from build123d import *

# Parameters (mm, degrees)
SKETCH_1_W          = 20
SKETCH_1_H          = 12
SKETCH_1_R          = 1.6
SKETCH_1_R_2        = 2.1
EXTRUDE_1_DEPTH     = 5.3
EXTRUDE_2_DEPTH     = 1.5
SKETCH_1_5_R        = 1.6
EXTRUDE_3_DEPTH     = 4
EXTRUDE_START       = 5.3
EXTRUDE_4_DEPTH     = 4.5
SKETCH_2_R          = 0.9
SKETCH_2_R_2        = 0.7
CUT_EXTRUDE_1_DEPTH = 26.299011838
CUT_EXTRUDE_START   = 9.8
SKETCH_2_3_R        = 1.5
CUT_EXTRUDE_2_DEPTH = 8.8
SKETCH_2_4_R        = 1
CUT_EXTRUDE_3_DEPTH = 7.8
SKETCH_2_5_R        = 0.3
CUT_EXTRUDE_4_DEPTH = 6


with BuildPart() as part:
    # 草图1 → 凸台-拉伸1 (new body)
    with BuildSketch(Plane(origin=(0, 0, 0), x_dir=(1, 0, 0), z_dir=(0, 1, 0))):
        with Locations((10, -6)):
            Rectangle(SKETCH_1_W, SKETCH_1_H)
        with BuildLine():
            ThreePointArc((12.439835428, -3.613463312), (18.220575086, -7.370363498), (11.50515478, -5.81011348))
            ThreePointArc((11.50515478, -5.81011348), (7.454652656, -2.789434091), (12.439835428, -3.613463312))
        make_face(mode=Mode.SUBTRACT)
        with Locations(Location((7.678736094, -8.970584613, 0), (0, 0, 270))):
            Circle(SKETCH_1_R, mode=Mode.SUBTRACT)
        with Locations(Location((5, -6, 0), (0, 0, 270))):
            Circle(SKETCH_1_R_2, mode=Mode.SUBTRACT)
    extrude(amount=EXTRUDE_1_DEPTH)

    # 草图1<4> → 凸台-拉伸2 (add)
    with BuildSketch(Plane(origin=(0, 0, 0), x_dir=(1, 0, 0), z_dir=(0, 1, 0))):
        with BuildLine():
            ThreePointArc((11.50515478, -5.81011348), (11.779424914, -4.629636502), (12.439835428, -3.613463312))
            ThreePointArc((12.439835428, -3.613463312), (7.454652656, -2.789434091), (11.50515478, -5.81011348))
        make_face()
    extrude(amount=EXTRUDE_2_DEPTH)

    # 草图1<5> → 凸台-拉伸3 (add)
    with BuildSketch(Plane(origin=(0, 0, 0), x_dir=(1, 0, 0), z_dir=(0, 1, 0))):
        with Locations(Location((7.678736094, -8.970584613, 0), (0, 0, 270))):
            Circle(SKETCH_1_5_R)
    extrude(amount=EXTRUDE_3_DEPTH)

    # 草图1<6> → 凸台-拉伸4 (add)
    with BuildSketch(Plane(origin=(0, 0, 0), x_dir=(1, 0, 0), z_dir=(0, 1, 0)).offset(EXTRUDE_START)):
        with BuildLine():
            Line((7.958677072, 0), (0, 0))
            Line((0, 0), (0, -12))
            Line((0, -12), (5.925840657, -12))
            ThreePointArc((5.925840657, -12), (4.429268792, -10.270954659), (4.319841502, -7.986802561))
            ThreePointArc((4.319841502, -7.986802561), (3.000111311, -5.359340003), (5.600909971, -3.987810345))
            ThreePointArc((5.600909971, -3.987810345), (6.188678117, -1.644412009), (7.958677072, 0))
        make_face()
        with BuildLine():
            Line((20, 0), (11.735482653, 0))
            ThreePointArc((11.735482653, 0), (12.869036074, -0.819060885), (13.675372646, -1.961700559))
            ThreePointArc((13.675372646, -1.961700559), (18.910698319, -7.664012819), (11.171707216, -7.845717845))
            ThreePointArc((11.171707216, -7.845717845), (11.090844977, -7.871351024), (11.009487245, -7.895365208))
            ThreePointArc((11.009487245, -7.895365208), (10.945672327, -10.226422042), (9.43163153, -12))
            Line((9.43163153, -12), (20, -12))
            Line((20, -12), (20, 0))
        make_face()
    extrude(amount=EXTRUDE_4_DEPTH)

    # 草图2 → 切除-拉伸1 (cut, through all)
    with BuildSketch(Plane(origin=(0, 0, 0), x_dir=(1, 0, 0), z_dir=(0, 1, 0))):
        with Locations(Location((2.3, -2.214171161, 0), (0, 0, 270))):
            Circle(SKETCH_2_R)
        with Locations(Location((7.7, -9.785828839, 0), (0, 0, 313.840961576))):
            Circle(SKETCH_2_R)
        with Locations(Location((11.5, -1.5, 0), (0, 0, 171.097944201))):
            Circle(SKETCH_2_R_2)
        with Locations(Location((18.5, -10.5, 0), (0, 0, 270))):
            Circle(SKETCH_2_R_2)
        with Locations(Location((18.5, -1.5, 0), (0, 0, 270))):
            Circle(SKETCH_2_R_2)
        with Locations(Location((11.5, -10.5, 0), (0, 0, 132.232284036))):
            Circle(SKETCH_2_R_2)
    extrude(amount=CUT_EXTRUDE_1_DEPTH, mode=Mode.SUBTRACT)

    # 草图2<3> → 切除-拉伸2 (cut)
    with BuildSketch(Plane(origin=(0, 0, 0), x_dir=(1, 0, 0), z_dir=(0, 1, 0)).offset(CUT_EXTRUDE_START)):
        with Locations(Location((2.3, -2.214171161, 0), (0, 0, 270))):
            Circle(SKETCH_2_3_R)
        with Locations(Location((7.7, -9.785828839, 0), (0, 0, 270))):
            Circle(SKETCH_2_3_R)
    extrude(amount=-CUT_EXTRUDE_2_DEPTH, mode=Mode.SUBTRACT)

    # 草图2<4> → 切除-拉伸3 (cut)
    with BuildSketch(Plane(origin=(0, 0, 0), x_dir=(1, 0, 0), z_dir=(0, 1, 0)).offset(CUT_EXTRUDE_START)):
        with Locations((11.5, -1.5)):
            Circle(SKETCH_2_4_R)
        with Locations(Location((18.5, -10.5, 0), (0, 0, 270))):
            Circle(SKETCH_2_4_R)
        with Locations(Location((18.5, -1.5, 0), (0, 0, 270))):
            Circle(SKETCH_2_4_R)
        with Locations(Location((11.5, -10.5, 0), (0, 0, 270))):
            Circle(SKETCH_2_4_R)
    extrude(amount=-CUT_EXTRUDE_3_DEPTH, mode=Mode.SUBTRACT)

    # 草图2<5> → 切除-拉伸4 (cut)
    with BuildSketch(Plane(origin=(0, 0, 0), x_dir=(1, 0, 0), z_dir=(0, 1, 0)).offset(CUT_EXTRUDE_START)):
        with Locations(Location((1.5, -6, 0), (0, 0, 270))):
            Circle(SKETCH_2_5_R)
        with Locations(Location((16.5, -1.1, 0), (0, 0, 270))):
            Circle(SKETCH_2_5_R)
        with Locations(Location((15, -10.9, 0), (0, 0, 270))):
            Circle(SKETCH_2_5_R)
    extrude(amount=-CUT_EXTRUDE_4_DEPTH, mode=Mode.SUBTRACT)


solid = part.part
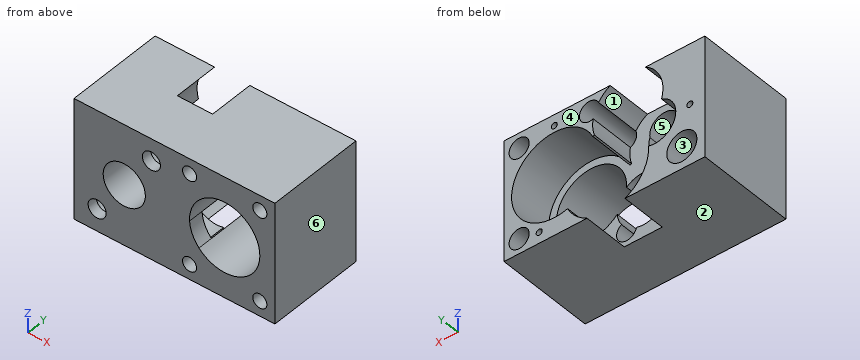
Source: CAD feature listing. Evaluate the final solid. Frame: model axes, mm. Face numbers are marked on the shaded views. A direction names the side the tool comes from. Round coordinates to 2 decimals unless told otherwise and drop trailing zeros. Write each loop counter-clockwise with the first axis right and the second up, starting at its lowest first coordinate (ties: lowest second). Pieces come first, ordered by that corner, then holes. Notation, with made-up numbers: (69.25, 80.5) - (114.25, 80.5) arc R7 cw to (114.25, 89.5) - close; hole circle Ø2 at (54.25, 35). An arc over 180 degrees is marked (long way). Use CSV: the item, a comma, the result in double quotes. Start each with the question number.
(1) Cut plane C-C, the plane z = 9.25. Return loops of the section in (x, y).
(2) Cut plane A-A, the plane y = 8.75. Return loops of the section in (x, z).
(3) Cut plane B-B, the plane x = 2.3. Return loops of the section in (y, z).
(4) Mould query, pull axis X, two halves, no side actions, for the marked faces 4, 5 and 6. Classes: pulls with the +X half, pulls with the -X half, needs draft (parallel to the pull), parting line crosses it, or undercut.
(5) First-contact query: pin 1 Ø1.8 at (x, z) = (11.5, 10.5) entering from +Y; pin 2 Ø5 at (x, z) = (8.5, 4.5) entering from +Y. Flat tips, straight axial feed; report the tip coordinate or a pass-through.
(6) Material intervals for probe 1 along Z at (x, y) = (16.5, 5.2); probe 2 along X at (y, z) = (1.45, 10.5); probe 3 along X at (y, z) = (5.75, 6.25), sorted ascending. Write a range as [from, to].
(7) Cut plane D-D, the plane x = 15. Return loops of the section in (y, z).
(8) Set-up query: the marked faces 1, 2 and 3. Return all of +Z, -Z, +X, -X, +Y, -Y with unobstructed straight access to the full face (end or side cutting, diameter ignored); none if empty.
Geometry says:
1,outline,"(0, 0) - (6.98, 0) - (6.98, 1) - (6.3, 1) - (6.3, 4) - (6.1, 4) - (6.1, 5.3) - (4.19, 5.3) - (4.19, 9.8) - (0, 9.8) - close; (8.42, 0) - (13.7, 0) - (13.7, 5.3) - (12.26, 5.3) - (12.26, 9.8) - (11.17, 9.8) - (11.17, 5.3) - (9.25, 5.3) - (9.25, 4) - (9.1, 4) - (9.1, 1) - (8.42, 1) - close; (16.3, 0) - (20, 0) - (20, 9.8) - (17.74, 9.8) - (17.74, 5.3) - (16.3, 5.3) - close"
2,outline,"(0, 0) - (7.96, 0) arc R4.25 cw to (5.6, 3.99) arc R2.1 cw to (4.32, 7.99) arc R3.5 cw to (5.93, 12) - (0, 12) - close; (9.43, 12) arc R3.5 cw to (10.59, 10.91) arc R1 cw (long way) to (11.13, 9.57) arc R3.5 cw to (11.01, 7.9) arc R4.25 cw to (11.17, 7.85) arc R4.25 cw (long way) to (13.68, 1.96) arc R4.25 cw to (11.74, 0) - (20, 0) - (20, 12) - close; hole circle Ø3 at (2.3, 2.21); hole circle Ø0.6 at (1.5, 6); hole circle Ø0.6 at (15, 10.9); hole circle Ø0.6 at (16.5, 1.1); hole circle Ø2 at (18.5, 1.5); hole circle Ø2 at (18.5, 10.5)"
3,outline,"(0, 0) - (9.8, 0) - (9.8, 0.71) - (1, 0.71) - (1, 1.31) - (0, 1.31) - close; (0, 3.11) - (1, 3.11) - (1, 3.71) - (9.8, 3.71) - (9.8, 12) - (0, 12) - close"
4,face 4,"needs draft"
4,face 5,"undercut"
4,face 6,"pulls with the +X half"
5,pin 1,"y = 2"
5,pin 2,"y = 5.3"
6,probe 1,"[0, 0.8], [1.4, 2.84], [9.16, 12]"
6,probe 2,"[0, 6.38], [9.02, 10.8], [12.2, 17.8], [19.2, 20]"
6,probe 3,"[0, 1.33], [1.67, 2.91], [19.24, 20]"
7,outline,"(0, 0) - (9.8, 0) - (9.8, 1.75) - (5.3, 1.75) - (5.3, 2.5) - (0, 2.5) - close; (0, 9.5) - (5.3, 9.5) - (5.3, 10.25) - (9.8, 10.25) - (9.8, 10.6) - (3.8, 10.6) - (3.8, 11.2) - (9.8, 11.2) - (9.8, 12) - (0, 12) - close"
8,face 1,"-Z, +Y"
8,face 2,"-Z, +X, -X, +Y, -Y"
8,face 3,"+Y"
